```python
from build123d import *

# Parameters (mm, degrees)
BOSS_EXTRUDE1_START = 17.5
SKETCH1_R           = 34.5
SKETCH1_R_2         = 32
BOSS_EXTRUDE1_DEPTH = 50
CHAMFER1_SIZE       = 0.5


with BuildPart() as part:
    # Sketch1 → Boss-Extrude1 (new body)
    with BuildSketch(Plane.XY.offset(BOSS_EXTRUDE1_START)):
        Circle(SKETCH1_R)
        Circle(SKETCH1_R_2, mode=Mode.SUBTRACT)
    extrude(amount=-BOSS_EXTRUDE1_DEPTH)

    # Chamfer1
    chamfer1_edges = [part.edges().sort_by_distance(p)[0] for p in [
        (-34.5, 0, 17.5),
        (-32, 0, 17.5),
        (-34.5, 0, -32.5),
        (-32, 0, -32.5),
    ]]
    chamfer(chamfer1_edges, length=CHAMFER1_SIZE)


solid = part.part
```
The listing builds one solid part. Answer for the finished solid, in the listing's coordinates (mm). Coordinates: 2 decimals unless noted, no trailing zeros. Write each loop counter-clockwise with the first axis right and the second up, starting at its lowest first coordinate (ties: lowest second). Pieces come first, ordered by that corner, then holes. Notation, with made-up numbers: (83, 9) - (137, 9) arc R22 cw to (137, 32) - close; hole circle Ø11 at (52.25, 29). An arc over 180 degrees is marked (long way). Return JSON: item names as keys, results as strings. Group by question number.
Q1. For a pull along X with two mould halves and no side action, classify faces 1 (the flat face through (28, -17, 17.5)), 2 (the cylindrical face through (32.907, 10.363, -7.157)), 3 (the cylindrical face through (-6.94, -31.24, -7.16)) as +X half, -X half, draft (parallel to the pull), parting line (faces both ways), or undercut.
Q2. The part is cut by section C-C on z = -5. Write down the section's boundary in (x, y), and give its area (3 significant figures).
Q3. Flat-ended cylindrical pins translate along their axes: pin 1 Ø4 at (y, z) = (3, -27) entering from -X; pin 2 Ø8 at (x, z) = (10.5, -9.5) entering from -Y; pin 3 Ø3 at (x, z) = (6.5, -4.5) entering from +Y; pin 4 Ø10 at (x, y) = (24, 24.5) entering from -Z. Find the tip coordinate at first contact, or state that the pin passes through.
Q4. The part is cut by section A-A on y = 0. Write down the section's boundary in (x, z), and give its area (3 significant figures).
Q5. Find the intervals of material crossed by line 1 along Y through (x, z) = (0, -7); line 2 along X through (y, z) = (1, -13); line 3 along X through (y, z) = (21.5, -24), in increasing order. Write a range as [from, to].
Evaluation:
{
 "1": {"face 1": "draft", "face 2": "parting line", "face 3": "undercut"},
 "2": {"outline": "circle Ø69 at (0, 0); hole circle Ø64 at (0, 0)", "area": "522 mm2"},
 "3": {"pin 1": "stops at x = -34.49", "pin 2": "stops at y = -33.88", "pin 3": "stops at y = 34.14", "pin 4": "stops at z = -32.5"},
 "4": {"outline": "(-34.5, -32) - (-34, -32.5) - (-32.5, -32.5) - (-32, -32) - (-32, 17) - (-32.5, 17.5) - (-34, 17.5) - (-34.5, 17) - close; (32, -32) - (32.5, -32.5) - (34, -32.5) - (34.5, -32) - (34.5, 17) - (34, 17.5) - (32.5, 17.5) - (32, 17) - close", "area": "249 mm2"},
 "5": {"line 1": "y = [-34.5, -32], [32, 34.5]", "line 2": "x = [-34.49, -31.98], [31.98, 34.49]", "line 3": "x = [-26.98, -23.7], [23.7, 26.98]"}
}
